from build123d import *

# Parameters (mm, degrees)
ESQUISSE1_W             = 680
ESQUISSE1_H             = 670
BOSS_EXTRU_1_DEPTH      = 10
ESQUISSE2_W             = 80
ESQUISSE2_H             = 30
ENL_V_MAT_EXTRU_1_DEPTH = 11
ESQUISSE3_W             = 52
ESQUISSE3_H             = 6
ENL_V_MAT_EXTRU_2_DEPTH = 11
ESQUISSE4_R             = 4
ENL_V_MAT_EXTRU_3_DEPTH = 11
ESQUISSE5_R             = 2
ENL_V_MAT_EXTRU_4_DEPTH = 11
ESQUISSE6_W             = 44
ESQUISSE6_H             = 71
ENL_V_MAT_EXTRU_5_DEPTH = 11
ENL_V_MAT_EXTRU_6_DEPTH = 11


with BuildPart() as part:
    # Esquisse1 → Boss.-Extru.1 (new body)
    with BuildSketch(Plane.XY):
        Rectangle(ESQUISSE1_W, ESQUISSE1_H)
    extrude(amount=BOSS_EXTRU_1_DEPTH)

    # Esquisse2 → Enlèv. mat.-Extru.1 (cut, through all)
    with BuildSketch(Plane.XY.offset(10)):
        with Locations((-300, 320)):
            Rectangle(ESQUISSE2_W, ESQUISSE2_H)
        with Locations((300, 320)):
            Rectangle(ESQUISSE2_W, ESQUISSE2_H)
    extrude(amount=-ENL_V_MAT_EXTRU_1_DEPTH, mode=Mode.SUBTRACT)

    # Esquisse3 → Enlèv. mat.-Extru.2 (cut, through all)
    with BuildSketch(Plane.XY.offset(10)):
        with Locations((-209.5, -293)):
            Rectangle(ESQUISSE3_W, ESQUISSE3_H)
    extrude(amount=-ENL_V_MAT_EXTRU_2_DEPTH, mode=Mode.SUBTRACT)

    # Esquisse4 → Enlèv. mat.-Extru.3 (cut, through all)
    with BuildSketch(Plane.XY.offset(10)):
        with Locations((-222, -315)):
            Circle(ESQUISSE4_R)
        with Locations((-197, -315)):
            Circle(ESQUISSE4_R)
    extrude(amount=-ENL_V_MAT_EXTRU_3_DEPTH, mode=Mode.SUBTRACT)

    # Esquisse5 → Enlèv. mat.-Extru.4 (cut, through all)
    with BuildSketch(Plane.XY.offset(10)):
        with Locations((-250, -266)):
            Circle(ESQUISSE5_R)
        with Locations((-169, -266)):
            Circle(ESQUISSE5_R)
    extrude(amount=-ENL_V_MAT_EXTRU_4_DEPTH, mode=Mode.SUBTRACT)

    # Esquisse6 → Enlèv. mat.-Extru.5 (cut, through all)
    with BuildSketch(Plane.XY.offset(10)):
        with Locations((-318, 229.5)):
            Rectangle(ESQUISSE6_W, ESQUISSE6_H)
    extrude(amount=-ENL_V_MAT_EXTRU_5_DEPTH, mode=Mode.SUBTRACT)

    # Esquisse7 → Enlèv. mat.-Extru.6 (cut, through all)
    with BuildSketch(Plane.XY.offset(10)):
        with BuildLine():
            Line((-246, 260), (-246, 240))
            ThreePointArc((-246, 240), (-244, 238), (-242, 240))
            Line((-242, 240), (-242, 260))
            ThreePointArc((-242, 260), (-244, 262), (-246, 260))
        make_face()
        with BuildLine():
            Line((-246, 219), (-246, 199))
            ThreePointArc((-246, 199), (-244, 197), (-242, 199))
            Line((-242, 199), (-242, 219))
            ThreePointArc((-242, 219), (-244, 221), (-246, 219))
        make_face()
    extrude(amount=-ENL_V_MAT_EXTRU_6_DEPTH, mode=Mode.SUBTRACT)


solid = part.part
Source: CAD feature listing. Evaluate the final solid. Frame: model axes, mm. Coordinates: 2 decimals unless noted, no trailing zeros. Loops run counter-clockwise (first coordinate to the right, second up) from the corner with the lowest first, then second, coordinate; pieces in that order, holes last. Notation, with made-up numbers: (23, 18) - (70, 18) arc R11 cw to (70, 30) - close; hole circle Ø1 at (33.25, 32). An arc over 180 degrees is marked (long way). One line per question, with ' | ' between items.
1) Line query: line 1 along X through (y, z) = (-315, 5.25); line 2 along Y through (x, z) = (-211, 4.5); line 3 along X through (y, z) = (-266, 2). Output: solid intervals per line, ascending.
Report:
line 1: x = -340 to -226, -218 to -201, -193 to 340 | line 2: y = -335 to -296, -290 to 335 | line 3: x = -340 to -252, -248 to -171, -167 to 340
2) Section A-A, the plane z = 8.25. Return loops of the section in (x, y), then the cut area to 3 significant figures.
Report:
outline: (-340, -335) - (340, -335) - (340, 305) - (260, 305) - (260, 335) - (-260, 335) - (-260, 305) - (-340, 305) - (-340, 265) - (-296, 265) - (-296, 194) - (-340, 194) - close; hole circle Ø4 at (-250, -266); hole (-246, 199) arc R2 ccw to (-242, 199) - (-242, 219) arc R2 ccw to (-246, 219) - close; hole (-246, 240) arc R2 ccw to (-242, 240) - (-242, 260) arc R2 ccw to (-246, 260) - close; hole (-235.5, -296) - (-183.5, -296) - (-183.5, -290) - (-235.5, -290) - close; hole circle Ø8 at (-222, -315); hole circle Ø8 at (-197, -315); hole circle Ø4 at (-169, -266) | area: 447,000 mm²
3) First-contact query: P1, Ø2.5, axis at x = -169, y = -266, coming from the -Z side; P2, Ø5, axis at y = 213, z = 5, coming from the -X side; P3, Ø5, axis at x = 299, z = 4.5, coming from the +Y side. Flat tips, straight axial feed; report the tip coordinate or a pass-through.
Report:
P1: passes through | P2: stops at x = -296 | P3: stops at y = 305
